Read the model definition and answer for the solid it produces. Units are mm, in the model's axes. Give positions to 0.01 mm unless a question says otherwise; leave off trailing zeros. Write each loop counter-clockwise with the first axis right and the second up, starting at its lowest first coordinate (ties: lowest second). Pieces come first, ordered by that corner, then holes.
```python
from build123d import *

# Parameters (mm, degrees)
SKETCH1_R           = 2.5
BOSS_EXTRUDE1_DEPTH = 5
SKETCH2_R           = 40
CUT_EXTRUDE1_DEPTH  = 2
CHAMFER1_SIZE       = 2.5


with BuildPart() as part:
    # Sketch1 → Boss-Extrude1 (new body)
    with BuildSketch(Plane(origin=(0, 0, 0), x_dir=(1, 0, 0), z_dir=(0, 1, 0))):
        with BuildLine():
            Line((-110, -53), (110, -53))
            ThreePointArc((110, -53), (163, 0), (110, 53))
            Line((110, 53), (-110, 53))
            ThreePointArc((-110, 53), (-163, 0), (-110, -53))
        make_face()
        with Locations((-110, -35)):
            Circle(SKETCH1_R, mode=Mode.SUBTRACT)
        with Locations((-110, 35)):
            Circle(SKETCH1_R, mode=Mode.SUBTRACT)
        with Locations((-79.689110868, 17.5)):
            Circle(SKETCH1_R, mode=Mode.SUBTRACT)
        with Locations((-79.689110868, -17.5)):
            Circle(SKETCH1_R, mode=Mode.SUBTRACT)
        with Locations((-140.310889132, 17.5)):
            Circle(SKETCH1_R, mode=Mode.SUBTRACT)
        with Locations((-140.310889132, -17.5)):
            Circle(SKETCH1_R, mode=Mode.SUBTRACT)
    extrude(amount=BOSS_EXTRUDE1_DEPTH)

    # Sketch2 → Cut-Extrude1 (cut)
    with BuildSketch(Plane(origin=(0, 5, 0), x_dir=(1, 0, 0), z_dir=(0, 1, 0))):
        with Locations((-110, 0)):
            Circle(SKETCH2_R)
    extrude(amount=-CUT_EXTRUDE1_DEPTH, mode=Mode.SUBTRACT)

    # Chamfer1
    chamfer1_edges = [part.edges().sort_by_distance(p)[0] for p in [
        (-163, 5, 0),
        (0, 5, 53),
        (163, 5, 0),
        (0, 5, -53),
    ]]
    chamfer(chamfer1_edges, length=CHAMFER1_SIZE)


solid = part.part
```
Item 1: Find the intervals of material crossed by line 1 along Z through (x, y) = (-110, 1.5); line 2 along X through (y, z) = (2.15, 16.5); line 3 along X through (y, z) = (0.7, -15.5), in increasing order.
Result set:
line 1: z = -53 to -37.5, -32.5 to 32.5, 37.5 to 53
line 2: x = -160.37 to -142.6, -138.02 to -81.98, -77.4 to 160.37
line 3: x = -160.68 to -141.81, -138.81 to -81.19, -78.19 to 160.68
Item 2: Each of these flat-tipped pins is pushed along its axis until it touches: pin 1 Ø3 at (y, z) = (2.5, 22) entering from -X; pin 2 Ø24 at (x, z) = (-91.5, -19) entering from +Y; pin 3 Ø3 at (y, z) = (4.5, -5) entering from -X; pin 4 Ø4.5 at (x, z) = (-79.69, -17.5) entering from -Y. Where does it stop, or does it pass through?
Result set:
pin 1: stops at x = -158.87
pin 2: stops at y = 3
pin 3: stops at x = -162.27
pin 4: passes through
Item 3: Section A-A (y = 4.1) is taken. Write down the section's boundary in (x, z), and give its area (3 significant figures).
Result set:
outline: (-110, -51.4) - (110, -51.4) arc R51.4 ccw to (110, 51.4) - (-110, 51.4) arc R51.4 ccw to start; hole circle Ø80 at (-110, 0)
area: 25,900 mm2
Item 4: Determine the mould class of faces 1 (the flat face through (-2, 0, -1)), 2 (the cylindrical face through (-71.847, 4.014, -12.015)), 3 (the flat face through (-111, 3, -1)), 4 (the conical face through (-160.61, 4.88, -1.11)) for opening direction Z: pulls with the +Z half, pulls with the -Z half, needs draft (parallel to the pull), parting line crosses it, or undercut.
Result set:
face 1: needs draft
face 2: undercut
face 3: undercut
face 4: parting line crosses it
Item 5: Section B-B (z = 0) is taken. Write down the section's boundary in (x, y), and give its area (3 significant figures).
Result set:
outline: (-163, 0) - (163, 0) - (163, 2.5) - (160.5, 5) - (-70, 5) - (-70, 3) - (-150, 3) - (-150, 5) - (-160.5, 5) - (-163, 2.5) - close
area: 1,460 mm2
